The figure shows three views and two pictorial views of one solid part (mm, origin at its lowest corner). Answer the questions. Round coordinates to 2 decimals unless told otherwise and drop trailing zeros. Loops run counter-clockwise (first coordinate to the right, second up) from the corner with the lowest first, then second, coordinate; pieces in that order, holes last. Notation, with made-up numbers: (59, 42) -> (66, 42) arc R19 cw to (66, 65) -> close; hole circle Ø7 at (28, 58.25). An arc over 180 degrees is marked (long way). Use a Markdown table: item, result. Add a question column.
Q1. Consider line 1 (X direction, y = 6, z = 82.5); line 2 (Z direction, x = 10, y = 3); line 3 (Z direction, x = 124, y = 7.5). Determine where each line is inside the solid, lowest interval first.
Q2. Section B-B on y = 3.75 is taken. Give the vertices of the cut face in (x, z).
Q3. Given pin 1 Ø5 at (y, z) = (3, 17) entering from -X; pin 2 Ø5 at (x, y) = (6.5, 4.5) entering from +Z; pin 3 Ø5 at (x, y) = (6, 3) entering from -Z, each flat-ended and moving along its own axis, determine where each tip first touches the part or whether it passes through.
Q4. Section C-C on x = 133.5 is taken. Give the vertices of the cut face in (y, z).
Q5. Section A-A on z = 77 is taken. Give the vertices of the cut face in (x, y).
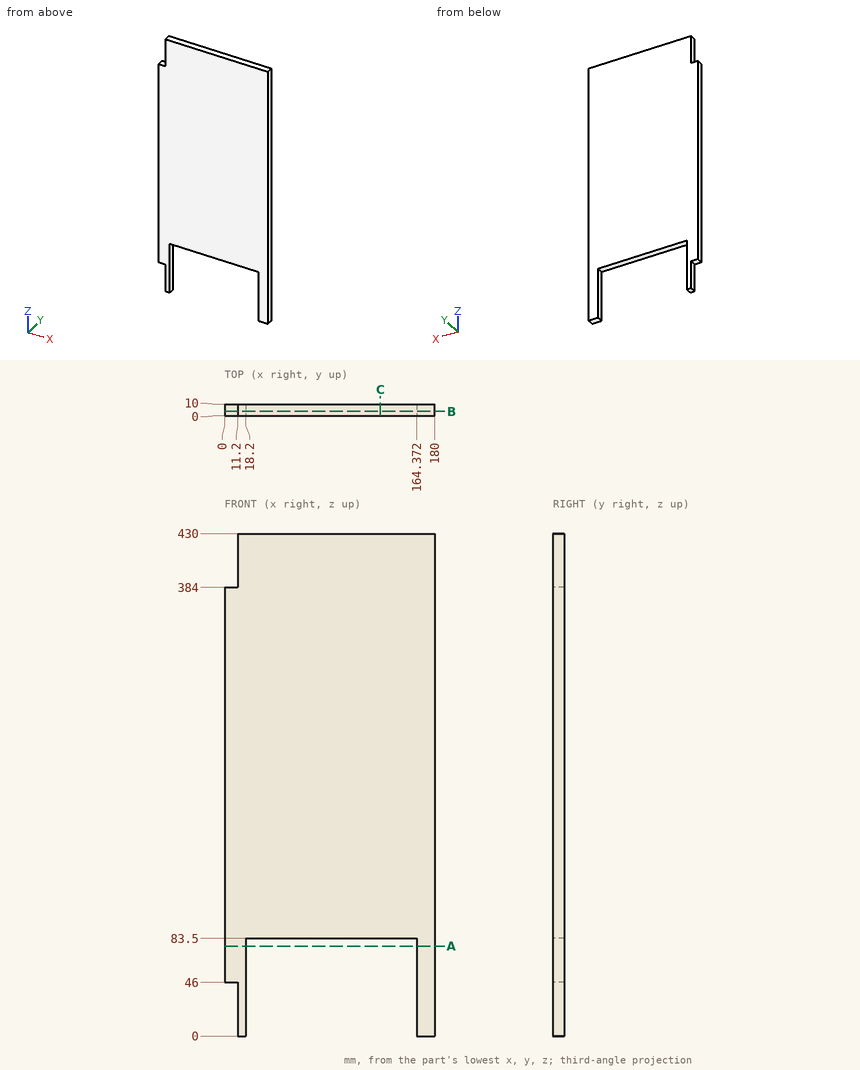
Checked values:
| question | item | result |
|---|---|---|
| 1 | line 1 | x = 0 to 18.2, 164.37 to 180 |
| 1 | line 2 | z = 46 to 384 |
| 1 | line 3 | z = 83.5 to 430 |
| 2 | outline | (0, 46) -> (11.2, 46) -> (11.2, 0) -> (18.2, 0) -> (18.2, 83.5) -> (164.37, 83.5) -> (164.37, 0) -> (180, 0) -> (180, 430) -> (11.2, 430) -> (11.2, 384) -> (0, 384) -> close |
| 3 | pin 1 | stops at x = 11.2 |
| 3 | pin 2 | stops at z = 384 |
| 3 | pin 3 | stops at z = 46 |
| 4 | outline | (0, 83.5) -> (10, 83.5) -> (10, 430) -> (0, 430) -> close |
| 5 | outline | (0, 0) -> (18.2, 0) -> (18.2, 10) -> (0, 10) -> close; (164.37, 0) -> (180, 0) -> (180, 10) -> (164.37, 10) -> close |
